Read the model definition and answer for the solid it produces. Units are mm, in the model's axes. A direction names the side the tool comes from. Give positions to 0.01 mm unless a question says otherwise; leave off trailing zeros. Write each loop counter-clockwise with the first axis right and the second up, starting at its lowest first coordinate (ties: lowest second). Pieces come first, ordered by that corner, then holes.
```python
from build123d import *

# Parameters (mm, degrees)
EXTRUDE_1_DEPTH      = 110
CUT_EXTRUDE_4_DEPTH  = 134.373777696
SKETCH_7_W           = 16.60831278
SKETCH_7_H           = 38.473598513
CUT_EXTRUDE_14_DEPTH = 134.373777696
SKETCH_8_W           = 5
SKETCH_8_H           = 30.968526609
EXTRUDE_2_DEPTH      = 110
SKETCH_10_W          = 5
SKETCH_10_H          = 26
EXTRUDE_4_DEPTH      = 110
SKETCH_16_W          = 45
SKETCH_16_H          = 4
EXTRUDE_7_DEPTH      = 110
FILLET_4_R           = 3
FILLET_5_R           = 6
SKETCH_18_W          = 113.67218818
SKETCH_18_H          = 61.649849458
CUT_EXTRUDE_18_DEPTH = 137.586229955
SKETCH_19_R          = 2.1
SKETCH_19_R_2        = 2
CUT_EXTRUDE_19_DEPTH = 143.431323365
SKETCH_22_W          = 25
SKETCH_22_H          = 3
EXTRUDE_10_DEPTH     = 50
FILLET_7_R           = 3
SKETCH_23_R          = 2
CUT_EXTRUDE_24_DEPTH = 10


with BuildPart() as part:
    # Эскиз1 → Бобышка-Вытянуть1 (new body)
    with BuildSketch(Plane(origin=(0, 0, 0), x_dir=(1, 0, 0), z_dir=(0, 1, 0))):
        Polygon((-66.825757576, 34.969739794), (-66.825757576, 29.969739794), (-63.825757576, 29.969739794), (-63.825757576, 31.969739794), (-38.825757576, 31.969739794), (-38.825757576, 6.969739794), (-63.825757576, 6.969739794), (-63.825757576, 8.969739794), (-66.825757576, 8.969739794), (-66.825757576, 3.969739794), (-22.123470102, 3.969739794), (-36.579007505, 34.969739794), align=None)
    extrude(amount=EXTRUDE_1_DEPTH)

    # Эскиз3 → Вырез-Вытянуть4 (cut, through all)
    with BuildSketch(Plane.XZ):
        Polygon((-66.825757576, -3.969739794), (-65.325757576, -8.969739794), (-66.825757576, -8.969739794), align=None)
        Polygon((-66.825757576, -29.969739794), (-66.825757576, -34.969739794), (-65.325757576, -29.969739794), align=None)
    extrude(amount=-CUT_EXTRUDE_4_DEPTH, mode=Mode.SUBTRACT)

    # Эскиз7 → Вырез-Вытянуть14 (cut, through all)
    with BuildSketch(Plane(origin=(0, 0, 0), x_dir=(-1, 0, 0), z_dir=(0, -1, 0))):
        with Locations((27.703474463, 20.539743139)):
            Rectangle(SKETCH_7_W, SKETCH_7_H)
    extrude(amount=-CUT_EXTRUDE_14_DEPTH, mode=Mode.SUBTRACT)

    # Эскиз8 → Бобышка-Вытянуть2 (add)
    with BuildSketch(Plane(origin=(0, 0, 0), x_dir=(-1, 0, 0), z_dir=(0, -1, 0))):
        with Locations((36.298943925, 19.454003098)):
            Rectangle(SKETCH_8_W, SKETCH_8_H)
    extrude(amount=-EXTRUDE_2_DEPTH)

    # Эскиз10 → Бобышка-Вытянуть4 (add)
    with BuildSketch(Plane.XZ):
        with Locations((-36.298943925, 9.030260206)):
            Rectangle(SKETCH_10_W, SKETCH_10_H)
    extrude(amount=-EXTRUDE_4_DEPTH)

    # Эскиз16 → Бобышка-Вытянуть7 (add, through all)
    with BuildSketch(Plane(origin=(0, 110, 0), x_dir=(1, 0, 0), z_dir=(0, 1, 0))):
        with Locations((-16.298943925, -24.030260206)):
            Rectangle(SKETCH_16_W, SKETCH_16_H)
    extrude(amount=-EXTRUDE_7_DEPTH)

    # Скругление4
    fillet_4_edges = [part.edges().sort_by_distance(p)[0] for p in [
        (-38.798943925, 55, -3.969739794),
        (-33.798943925, 55, 22.030260206),
    ]]
    fillet(fillet_4_edges, radius=FILLET_4_R)

    # Скругление5
    fillet_5_edges = [part.edges().sort_by_distance(p)[0] for p in [
        (-38.798943925, 55, 26.030260206),
    ]]
    fillet(fillet_5_edges, radius=FILLET_5_R)

    # Эскиз18 → Вырез-Вытянуть18 (cut, through all)
    with BuildSketch(Plane(origin=(6.201056075, 0, 0), x_dir=(0, 0, -1), z_dir=(1, 0, 0))):
        with Locations((3.709673157, 29.175075271)):
            Rectangle(SKETCH_18_W, SKETCH_18_H)
    extrude(amount=-CUT_EXTRUDE_18_DEPTH, mode=Mode.SUBTRACT)

    # Эскиз19 → Вырез-Вытянуть19 (cut, through all)
    with BuildSketch(Plane(origin=(0, 0, -34.969739794), x_dir=(-1, 0, 0), z_dir=(0, 0, -1))):
        with Locations((51.70238254, 85)):
            Circle(SKETCH_19_R)
        with Locations((3.798943925, 85)):
            Circle(SKETCH_19_R_2)
    extrude(amount=-CUT_EXTRUDE_19_DEPTH, mode=Mode.SUBTRACT)

    # Эскиз22 → Бобышка-Вытянуть10 (add)
    with BuildSketch(Plane.XZ.offset(-60)):
        with Locations((-21.298943925, -30.469739794)):
            Rectangle(SKETCH_22_W, SKETCH_22_H)
    extrude(amount=-EXTRUDE_10_DEPTH)

    # Скругление7
    fillet_7_edges = [part.edges().sort_by_distance(p)[0] for p in [
        (-33.798943925, 85, -28.969739794),
    ]]
    fillet(fillet_7_edges, radius=FILLET_7_R)

    # Эскиз23 → Вырез-Вытянуть24 (cut)
    with BuildSketch(Plane(origin=(0, 0, -31.969739794), x_dir=(-1, 0, 0), z_dir=(0, 0, -1))):
        with Locations((21.298943925, 85)):
            Circle(SKETCH_23_R)
    extrude(amount=-CUT_EXTRUDE_24_DEPTH, mode=Mode.SUBTRACT)


solid = part.part
```
Item 1: Find the intervals of material crossed by line 1 along Z through (x, y) = (-22.5, 90); line 2 along Z through (x, y) = (-43, 80); line 3 along Z through (x, y) = (-21, 84), in increasing order.
Result set:
line 1: z = -31.97 to -28.97, 22.03 to 26.03
line 2: z = -34.97 to -31.97, -6.97 to -3.97
line 3: z = 22.03 to 26.03
Item 2: Determine the mould class of faces 5 (the flat face through (-13, 85, 22.03)), 6 (the flat face through (-35, 85, -34.938)), 7 (the flat face through (-63.826, 85, -31)), 8 (the cylindrical face through (-37.088, 84.65, 24.226)) for opening direction Z: pulls with the +Z half, pulls with the -Z half, needs draft (parallel to the pull), parting line crosses it, or undercut.
Result set:
face 5: undercut
face 6: pulls with the -Z half
face 7: undercut
face 8: pulls with the +Z half
Item 3: Each of these flat-tipped pins is pushed along its axis until it touches: pin 1 Ø1.5 at (y, z) = (96.5, -18.5) entering from +X; pin 2 Ø12.5 at (x, y) = (-18.5, 96) entering from -Z; pin 3 Ø1 at (y, z) = (99, 13.5) entering from -X. Where does it stop, or does it pass through?
Result set:
pin 1: stops at x = -33.8
pin 2: stops at z = -31.97
pin 3: stops at x = -38.8
Item 4: Section A-A (x = -47) is taken. Write down the section's boundary in (y, z).
Result set:
outline: (60, -34.97) - (110, -34.97) - (110, -31.97) - (60, -31.97) - close; (60, -6.97) - (110, -6.97) - (110, -3.97) - (60, -3.97) - close
Item 5: Section B-B (z = -8) is taken. Write down the section's boundary in (x, y), and give its area (3 significant figures).
Result set:
outline: (-65.62, 60) - (-63.83, 60) - (-63.83, 110) - (-65.62, 110) - close; (-38.83, 60) - (-33.8, 60) - (-33.8, 110) - (-38.83, 110) - close
area: 341 mm2
Item 6: Section D-D (y = 85) is taken. Give the number of separate pieces and of enclosed holes in the cut face, and give its area (3 significant figures).
Result set:
separate pieces: 5
enclosed holes: 0
area: 658 mm2
Item 7: Which of the six approach directions +Z, -Z, +X, -X, +Y, -Y give full straight-line access (tool end or side, diameter ignored) to faces 1 (the cylindrical face through (-21.039, 86.983, -30.491)), 2 (the flat face through (-33.799, 85, -4)), 3 (the flat face through (-54, 85, -3.97)), 4 (the flat face through (-38.826, 85, -20))?
Result set:
face 1: -Z
face 2: +X, +Y, -Y
face 3: +Z, -X, +Y, -Y
face 4: +Y, -Y
